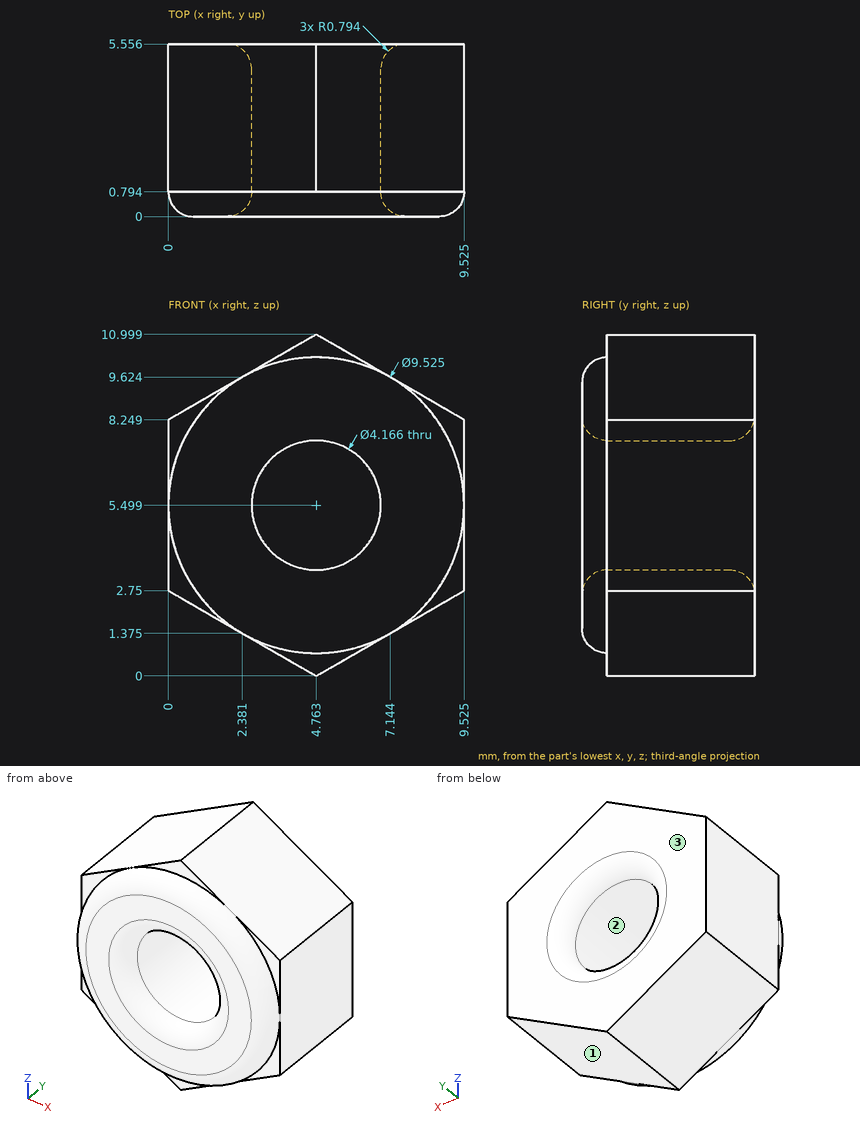
Study the drawing (mm; zero at the part's minimum x, y, z) and answer. Coordinates: 2 decimals unless noted, no trailing zeros. Return JSON: item names as keys, results as strings. Group by question number.
1. Straight lines are drawn through the part: L1, parallel to Z at x = 5.25, y = 1.25 (1 decimal); L2, parallel to X at y = 1.35, z = 5 (1 decimal); L3, parallel to Z at x = 4, y = 2.25. For each, find the intervals that lie inside material, in ascending order.
2. Given pin 1 (1.5 mm diameter, centred on x = 4, z = 10.5, fed in from -Y); pin 2 (3 mm diameter, centred on x = 5.5, z = 4.5, fed in from -Y), each flat-ended and moving along its own axis, determine where each tip first touches the part or whether it passes through.
3. Determine the mould class of the marked faces 1, 2 and 3 for opening direction Z: released by +Z, released by -Z, zero draft, split by the parting line, or undercut.
Ans:
{
 "1": {"L1": "0.3 to 3.5, 7.5 to 10.7", "L2": "0 to 2.7, 6.8 to 9.5", "L3": "0.44 to 3.56, 7.44 to 10.56"},
 "2": {"pin 1": "y = 0.08", "pin 2": "y = 0.01"},
 "3": {"face 1": "released by -Z", "face 2": "undercut", "face 3": "zero draft"}
}
